Design review of the part shown in the three views and the two pictorial views. Dimensions are in mm from the part's minimum x, y and z. Round coordinates to 2 decimals unless told otherwise and drop trailing zeros. Order: outer loops, then holes, each group sorted by start corner. A loop starts at its lowest first (then second) coordinate and runs counter-clockwise, first axis right, second up. Notation, with made-up numbers: M -9.5,3.25 L 21.5,3.25 A23 cw 21.5,22.25 Z; hole C -40,84 d11. An arc over 180 degrees is marked long. Use a Markdown table: item, result. Add a question column.
(1) To check wall thickness, follow probe 1 along Y at (x, z) = (240, 2.75); probe 2 along X at (y, z) = (4.5, 1); probe 3 along X at (y, z) = (14.5, 3.25). State the ranges of each line that lie inside material, in increasing order. Write a range as from..to.
(2) For pin 1 (1.5 mm diameter, centred on y = 9.5, z = 3.5, fed in from -X); pin 2 (5.5 mm diameter, centred on x = 126, y = 12.5, fed in from -Z), all flat-tipped, find the tip position at first contact; note any pin that passes through.
(3) Take a section at D-D (x = 240). Write out the cut boundary in (y, z), then the cut area to 3 significant figures.
(4) Take a section at C-C (z = 3.5). Write out the cut boundary in (x, y), then the cut area to 3 significant figures.
(5) Take a section at B-B (y = 12.5). Write out the cut boundary in (x, z), then the cut area to 3 significant figures.
(6) Take a section at A-A (x = 126). Write out the cut boundary in (y, z), then the cut area to 3 significant figures.
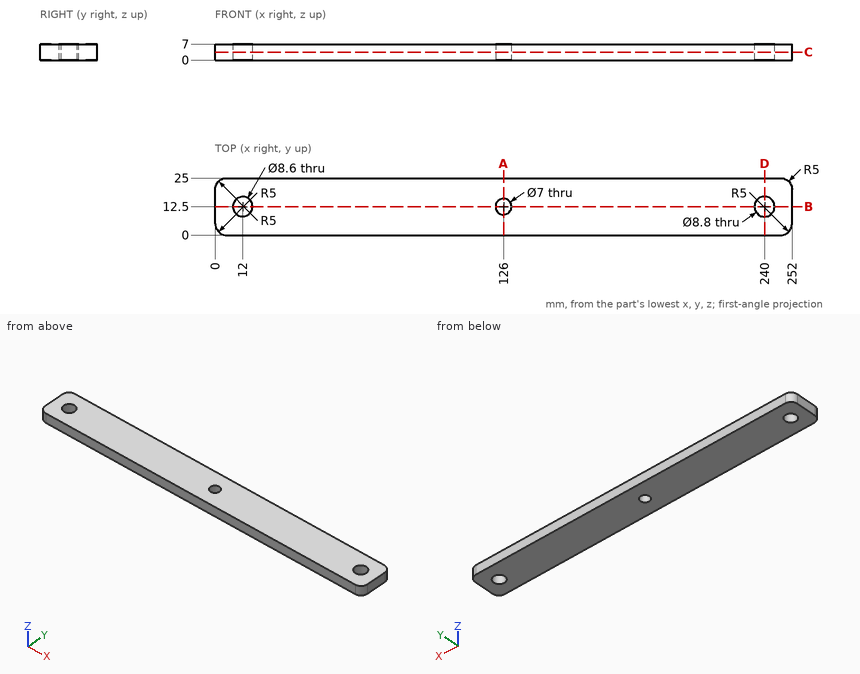
Verdict:
| question | item | result |
|---|---|---|
| 1 | probe 1 | y = 0..8.1, 16.9..25 |
| 1 | probe 2 | x = 0.03..251.97 |
| 1 | probe 3 | x = 0..8.19, 15.81..123.13, 128.87..236.08, 243.92..252 |
| 2 | pin 1 | stops at x = 0 |
| 2 | pin 2 | passes through |
| 3 | outline | M 0,0 L 8.1,0 L 8.1,7 L 0,7 Z; M 16.9,0 L 25,0 L 25,7 L 16.9,7 Z |
| 3 | area | 113 mm^2 |
| 4 | outline | M 0,5 A5 ccw 5,0 L 247,0 A5 ccw 252,5 L 252,20 A5 ccw 247,25 L 5,25 A5 ccw 0,20 Z; hole C 12,12.5 d8.6; hole C 126,12.5 d7; hole C 240,12.5 d8.8 |
| 4 | area | 6,120 mm^2 |
| 5 | outline | M 0,0 L 7.7,0 L 7.7,7 L 0,7 Z; M 16.3,0 L 122.5,0 L 122.5,7 L 16.3,7 Z; M 129.5,0 L 235.6,0 L 235.6,7 L 129.5,7 Z; M 244.4,0 L 252,0 L 252,7 L 244.4,7 Z |
| 5 | area | 1,590 mm^2 |
| 6 | outline | M 0,0 L 9,0 L 9,7 L 0,7 Z; M 16,0 L 25,0 L 25,7 L 16,7 Z |
| 6 | area | 126 mm^2 |
